The listing builds one solid part. Answer for the finished solid, in the listing's coordinates (mm). A direction names the side the tool comes from. Coordinates: 2 decimals unless noted, no trailing zeros. Write each loop counter-clockwise with the first axis right and the second up, starting at its lowest first coordinate (ties: lowest second). Pieces come first, ordered by that corner, then holes.
from build123d import *

# Parameters (mm, degrees)
BOSS_EXTRUDE1_DEPTH = 5
SKETCH4_W           = 2
SKETCH4_H           = 3
CUT_EXTRUDE3_DEPTH  = 15


with BuildPart() as part:
    # Sketch1 → Boss-Extrude1 (new body)
    with BuildSketch(Plane(origin=(0, 0, 0), x_dir=(1, 0, 0), z_dir=(0, 1, 0))):
        Polygon((4, 2), (4, 0), (0, 0), (0, 2), (0, 4), (6, 4), align=None)
    extrude(amount=BOSS_EXTRUDE1_DEPTH)

    # Sketch4 → Cut-Extrude3 (cut)
    with BuildSketch(Plane.ZY):
        with Locations((-1, 3.5)):
            Rectangle(SKETCH4_W, SKETCH4_H)
    extrude(amount=-CUT_EXTRUDE3_DEPTH, mode=Mode.SUBTRACT)


solid = part.part
1. A tool of negligible diameter and unlimited length cuts with its end or side. For faces 1 (the flat face through (4, 1, -1)), 2 (the flat face through (2, 2, -1)), 3 (the flat face through (0, 1.9, -2.5)), from which of +Z, -Z, +X, -X, +Y, -Y can it reach the whole face along a straight path? Write none if from no direction.
Results found:
face 1: +Z, +X, +Y, -Y
face 2: +Z, +X, -X, +Y
face 3: +Z, -Z, -X, +Y, -Y
2. Flat-ended cylindrical pins translate along their axes: P1, Ø0.9, axis at x = 1, y = 3, coming from the +Z side; P2, Ø1, axis at y = 3, z = -2.5, coming from the +X side; P3, Ø3, axis at x = 3, y = 2.5, coming from the +Z side; P4, Ø1, axis at x = 4, z = -0.5, coming from the +Y side. Find the tip coordinate at first contact, or state that the pin passes through.
Results found:
P1: stops at z = -2
P2: stops at x = 5
P3: stops at z = 0
P4: stops at y = 2
3. Section A-A on y = 0.9 is taken. Give the vertices of the cut face in (x, z).
Results found:
outline: (0, -4) - (6, -4) - (4, -2) - (4, 0) - (0, 0) - close
4. Find the intervals of material crossed by L1, parallel to X at y = 0.25, z = -1.6; L2, parallel to Z at x = 1.85, y = 2.75; L3, parallel to Y at x = 1.4, z = -0.35, in increasing order.
Results found:
L1: x = 0 to 4
L2: z = -4 to -2
L3: y = 0 to 2
5. Section C-C on z = -0.75 is taken. Give the vertices of the cut face in (x, y).
Results found:
outline: (0, 0) - (4, 0) - (4, 2) - (0, 2) - close
6. Section B-B on x = 3.2 is taken. Give the vertices of the cut face in (y, z).
Results found:
outline: (0, -4) - (5, -4) - (5, -2) - (2, -2) - (2, 0) - (0, 0) - close
7. Section D-D on z = -3.65 is taken. Give the vertices of the cut face in (x, y), then the cut area to 4 significant figures.
Results found:
outline: (0, 0) - (5.65, 0) - (5.65, 5) - (0, 5) - close
area: 28.25 mm2
